Input: part model. Units: mm. Frame: model coordinates. A direction names the side the tool comes from. Round coordinates to 2 decimals unless told otherwise and drop trailing zeros. Write each loop counter-clockwise with the first axis right and the second up, starting at its lowest first coordinate (ties: lowest second). Pieces come first, ordered by that corner, then holes. Notation, with made-up numbers: (-14, -32) - (8, -32) arc R13 cw to (8, -10) - close; hole circle Ø4 at (47.5, -36). An arc over 180 degrees is marked (long way). Use one line per item in the form item = value.
Autodesk Inventor part; units mm, degrees
ref_plane "YZ Plane" through (0, 0, 0) normal (1, 0, 0) x (0, 1, 0)
ref_plane "XZ Plane" through (0, 0, 0) normal (0, 1, 0) x (-1, 0, 0)
ref_plane "XY Plane" through (0, 0, 0) normal (0, 0, 1) x (1, 0, 0)
sketch "Sketch1" plane through (0, 0, 0) normal (0, 0, 1) x (1, 0, 0)
  line L0 (-21, 10) -> (21, 10)
  line L1 (21, 10) -> (21, -10)
  line L2 (21, -10) -> (-21, -10)
  line L3 (-21, -10) -> (-21, 10)
  line L4 (21, 15) -> (-19.3814, 15)
  line L5 (21, -15) -> (-21.3289, -15)
  arc A0 (-30.3889, 10.9551) -> (-106.2021, -86.7378) centre (164.8345, -218.8085) ccw
  arc A1 (-106.2021, -86.7378) -> (-103.2462, -89.2462) centre (-104.4035, -87.6142) ccw
  arc A2 (-30.3302, -17.5786) -> (-103.2462, -89.2462) centre (94.391, -217.3993) ccw
  arc A3 (-19.3814, 15) -> (-30.3889, 10.9551) centre (-19.3814, -2) ccw
  arc A4 (-21.3289, -15) -> (-30.3302, -17.5786) centre (-21.3289, -32) ccw
  arc A5 (21, -15) -> (21, 15) centre (14.4642, 0) ccw
  point P0 (0, 0)
  point P1 (-21, 0)
  point P2 (-26.1005, -15)
  point P3 (-25.5259, 15)
  dimension "d0" = 42
  dimension "d1" = 20
  dimension "d2" = 10
  dimension "d3" = 21
  dimension "d15" = 301.502
  dimension "d16" = 235.5497
  dimension "d17" = 17
extrude "Extrusion1" add sketch "Sketch1" along normal blind 40.5 contours L0 L1 L2 L3 | A5 L5 A4 A2 A1 A0 A3 L4
sketch "Sketch2" plane through (-19.3814, 15, 0) normal (0, 1, 0) x (1, 0, 0)
  line L0 (0, 0) -> (0, -40.5)
  line L1 (0, -20.25) -> (-86.8207, -20.25)
  line L2 (-86.8207, 0) -> (-86.8207, -40.5)
  line L3 (-11.0075, 0) -> (0, 0)
  line L4 (-11.0075, -40.5) -> (0, -40.5)
  line L5 (-83.8648, 0) -> (-83.8648, -40.5)
  line L6 (-83.8648, -20.25) -> (-83.8648, -23.206)
  line L7 (-83.8648, -23.206) -> (-11.0075, -40.5)
  line L8 (-87.0229, 0) -> (-87.0229, -40.5)
  arc A0 (-87.0229, -20.25) -> (-83.8648, -23.206) centre (-82.8584, -18.9658) ccw
  line L9 (-83.8648, -17.294) -> (-11.0075, 0)
  arc A1 (-83.8648, -17.294) -> (-87.0229, -20.25) centre (-82.8584, -21.5342) ccw
  line L10 (-11.0075, -40.5) -> (-87.0229, -40.5)
  line L11 (-11.0075, 0) -> (-87.0229, 0)
  line L12 (-87.0229, -40.5) -> (-87.0229, 0)
  point P0 (19.3814, 0)
  dimension "d19" = 2.956
extrude "Extrusion2" cut sketch "Sketch2" against normal through all contours L9 L5 L11 | A1 L2 L11 L5 | L10 L5 L7 | L5 L10 L2 A0 | A1 L8 L11 L2 | L2 L10 L8 A0
sketch "Sketch3" plane through (0, 0, 40.5) normal (0, 0, 1) x (1, 0, 0)
  line L0 (-21.3289, -15) -> (21, -15)
  line L1 (21, 15) -> (21, -15)
  line L2 (21, 0) -> (-21, 0)
  line L3 (-21, 0) -> (-21, 10)
  line L4 (-21, 10) -> (21, 10)
  line L5 (21, 10) -> (21, -10)
  line L6 (21, -10) -> (-21, -10)
  line L7 (-21, -10) -> (-21, 10)
  point P0 (0, 0)
  dimension "d22" = 42
  dimension "d23" = 10
  dimension "d24" = 42
  dimension "d25" = 20
extrude "Extrusion3" cut sketch "Sketch3" against normal blind 38.5
properties part number "Spider_Robot_Tibia_V1"
(1) Material intervals for L1, parallel to Y at x = -18, z = 8; L2, parallel to X at y = 1, z = 14.5; L3, parallel to Z at x = -8.5, y = 1, sorted ascending.
Derived:
L1 = -15 to -10, 10 to 15
L2 = -41.53 to -21, 21 to 30.8
L3 = 0 to 2
(2) Cut plane A-A on x = -9.5. Output: boundary loops of the cut face in (y, z), then the cut area to 3 significant figures.
Derived:
outline = (-15, 0) - (15, 0) - (15, 40.5) - (10, 40.5) - (10, 2) - (-10, 2) - (-10, 40.5) - (-15, 40.5) - close
area = 445 mm^2
(3) Access query for faces 1 (the face through (1, 15, 20)), 2 (the face through (0, -15, 20)), 3 (the face through (-21, 0, 22)). Directions: +Z, -Z, +X, -X, +Y, -Y. A direction counts if a zero-diameter tool reaches every point of the face in a straight line with its end or side. Return the directions, or none.
Derived:
face_1 = +Z, -Z, +X, -X, +Y
face_2 = +Z, -Z, +X, -Y
face_3 = +Z
(4) First-contact query: pin 1 Ø3 at (x, z) = (-34, 35.5) entering from +Y; pin 2 Ø1 at (x, z) = (-44, 7.5) entering from +Y; pin 3 Ø10 at (y, z) = (3, 20) entering from -X; pin 4 Ø1.5 at (x, y) = (-19, -16.5) entering from -Z. Flat tips, straight axial feed; report the tip coordinate or a pass-through.
Derived:
pin_1 = 9.14
pin_2 = -0.86
pin_3 = -44.68
pin_4 = through
(5) Cut plane C-C on y = 5. Output: boundary loops of the cut face in (x, z), then the cut area to 3 significant figures.
Derived:
outline = (-37.19, 1.61) - (-30.39, 0) - (30.04, 0) - (30.04, 40.5) - (21, 40.5) - (21, 2) - (-21, 2) - (-21, 40.5) - (-30.39, 40.5) - (-37.19, 38.89) - close
area = 1,090 mm^2
(6) Cut plane D-D on z = 34. Output: boundary loops of the cut face in (x, y).
Derived:
outline = (-57.77, -37.59) arc R235.55 cw to (-30.33, -17.58) arc R17 cw to (-21.33, -15) - (21, -15) arc R16.36 ccw to (21, 15) - (-19.38, 15) arc R17 ccw to (-30.39, 10.96) arc R301.5 ccw to (-57.77, -15.46) - close; hole (-21, -10) - (21, -10) - (21, 10) - (-21, 10) - close
(7) Cut plane B-B on z = 12. Output: boundary loops of the cut face in (x, y).
Derived:
outline = (-80.94, -60.1) arc R235.55 cw to (-30.33, -17.58) arc R17 cw to (-21.33, -15) - (21, -15) arc R16.36 ccw to (21, 15) - (-19.38, 15) arc R17 ccw to (-30.39, 10.96) arc R301.5 ccw to (-80.94, -44.18) - close; hole (-21, -10) - (21, -10) - (21, 10) - (-21, 10) - close
(8) Draft query along X for faces 4 (the face through (0, -1, 0)), 5 (the face through (0, 10, 22)), 6 (the face through (-61.591, -35.201, 33.094)), 7 (the face through (21, 0, 22)). Return one class per face: released by +X, released by -X, zero draft, split by the parting line, or undercut.
Derived:
face_4 = zero draft
face_5 = undercut
face_6 = released by -X
face_7 = undercut
